```python
from build123d import *

# Parameters (mm, degrees)
F1_DEPTH = 38.1
F2_R     = 6.35
F3_DEPTH = 12.7
F4_DEPTH = 12.7


with BuildPart() as f1:
    # F0 (on Front) → F1 (new body)
    with BuildSketch(Plane.XZ):
        with BuildLine():
            ThreePointArc((12.7, 25.4), (-8.980256, 34.380256), (0, 12.7))
            ThreePointArc((0, 12.7), (8.980256, 16.419744), (12.7, 25.4))
        make_face()
        with BuildLine():
            Line((-63.5, 12.7), (-63.5, 0))
            Line((-63.5, 0), (0, 0))
            Line((0, 0), (63.5, 0))
            Line((63.5, 0), (63.5, 12.7))
            Line((63.5, 12.7), (37.5412, 12.7))
            Line((37.5412, 12.7), (31.439186, 12.7))
            ThreePointArc((31.439186, 12.7), (22.45893, 16.419744), (18.739186, 25.4))
            ThreePointArc((18.739186, 25.4), (-0.155407, 46.878344), (-19.05, 25.4))
            ThreePointArc((-19.05, 25.4), (-22.769744, 16.419744), (-31.75, 12.7))
            Line((-31.75, 12.7), (-37.5412, 12.7))
            Line((-37.5412, 12.7), (-63.5, 12.7))
        make_face()
        with BuildLine():
            ThreePointArc((12.7, 25.4), (8.980256, 16.419744), (0, 12.7))
            ThreePointArc((0, 12.7), (-8.980256, 34.380256), (12.7, 25.4))
        make_face(mode=Mode.SUBTRACT)
    extrude(amount=F1_DEPTH)

    # F2 (on face) → F3 (cut, through all)
    with BuildSketch(Plane.XY.offset(12.7)):
        with Locations((-44.45, -19.05)):
            Circle(F2_R)
    extrude(amount=-F3_DEPTH, mode=Mode.SUBTRACT)

    # F2 (on face) → F4 (cut, through all)
    with BuildSketch(Plane.XY.offset(12.7)):
        with Locations((44.45, -19.05)):
            Circle(F2_R)
        with Locations((-44.45, -19.05)):
            Circle(F2_R)
    extrude(amount=-F4_DEPTH, mode=Mode.SUBTRACT)


solid = f1.part
```
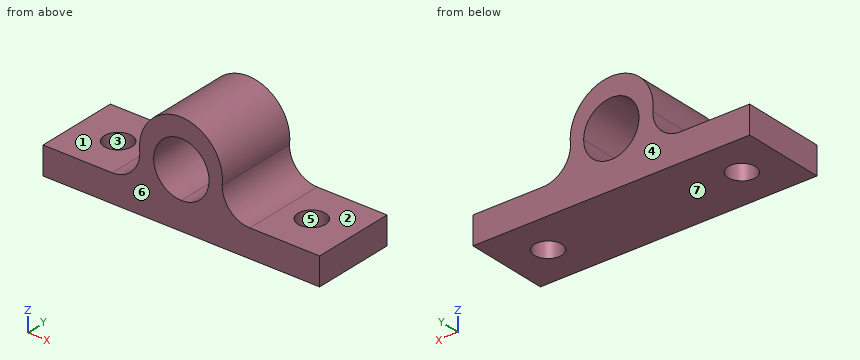
Here's how the part is built. I have some questions about the finished solid (model axes, mm). Face numbers are marked on the shaded views. A direction names the side the tool comes from. Give positions to 0.01 mm unless a question says otherwise; leave off trailing zeros. Write each loop counter-clockwise with the first axis right and the second up, starting at its lowest first coordinate (ties: lowest second). Pieces come first, ordered by that corner, then holes. Notation, with made-up numbers: M -19,47 L 16,47 A7 ccw 16,57 Z; hole C 56,-21 d10. An arc over 180 degrees is marked long. Put each result on its own line as item: value. Start each with the question number.
Item 1: If we section it at B-B, the plane x = -44.45: Write out the boundary of the cut face in (y, z), then the cut area to 3 significant figures.
Item 2: If we section it at D-D, the plane z = 20: Write out the boundary of the cut face in (x, y), then the cut area to 3 significant figures.
Item 3: I need wall thicknesses on L1, parallel to X at y = -19, z = 5; L2, parallel to Y at x = 44.45, z = 6; L3, parallel to X at y = -21.5, z = 4.5. Which ranges of each line are inside material? Lowest first, please. Write a range as from..to.
Item 4: Will these pins go through, and if not, where does the flat tip stop? pin 1 (1.5 mm diameter, centred on y = -24, z = 25, fed in from +X); pin 2 (8 mm diameter, centred on x = 29.5, y = -20, fed in from +Z); pin 3 (9.5 mm diameter, centred on x = 54, y = -12.5, fed in from +Z).
Item 5: If we section it at C-C, the plane y = -35: Write out the boundary of the cut face in (x, z).
Item 6: Thinking about a two-plate mould opening in Y: for the marked faces 4, 5, 6 and 7, which applies, +Y half, -Y half, draft (parallel to the pull), parting line (faces both ways), or undercut?
Item 7: On a 3-axis mill with a long thin cutter (end or side, diameter ignored), from which of +Z, -Z, +X, -X, +Y, -Y can I reach the whole of each face in a straight line? I mean the marked faces 1, 2 and 3. Say none if no direction works.
Item 8: If we section it at A-A, the plane y = -19.05: Write out the boundary of the cut face in (x, z), then the cut area to 3 significant figures.
Values:
1. outline: M -38.1,0 L -25.4,0 L -25.4,12.7 L -38.1,12.7 Z; M -12.7,0 L 0,0 L 0,12.7 L -12.7,12.7 Z
1. area: 323 mm²
2. outline: M -20.26,-38.1 L -11.49,-38.1 L -11.49,0 L -20.26,0 Z; M 11.49,-38.1 L 19.94,-38.1 L 19.94,0 L 11.49,0 Z
2. area: 656 mm²
3. L1: -63.5..-50.8, -38.1..38.1, 50.8..63.5
3. L2: -38.1..-25.4, -12.7..0
3. L3: -63.5..-50.31, -38.59..38.59, 50.31..63.5
4. pin 1: x = 18.79
4. pin 2: z = 14.17
4. pin 3: z = 12.7
5. outline: M -63.5,0 L 63.5,0 L 63.5,12.7 L 31.44,12.7 A12.7 cw 18.74,25.4 A19.05 ccw long -19.05,25.4 A12.7 cw -31.75,12.7 L -63.5,12.7 Z; hole C 0,25.4 d25.4
6. face 4: +Y half
6. face 5: undercut
6. face 6: -Y half
6. face 7: draft
7. face 1: +Z, -X, +Y, -Y
7. face 2: +Z, +X, +Y, -Y
7. face 3: +Z, -Z
8. outline: M -63.5,0 L -50.8,0 L -50.8,12.7 L -63.5,12.7 Z; M -38.1,0 L 38.1,0 L 38.1,12.7 L 31.44,12.7 A12.7 cw 18.74,25.4 A19.05 ccw long -19.05,25.4 A12.7 cw -31.75,12.7 L -38.1,12.7 Z; M 50.8,0 L 63.5,0 L 63.5,12.7 L 50.8,12.7 Z; hole C 0,25.4 d25.4
8. area: 2,000 mm²
